```python
from build123d import *

# Parameters (mm, degrees)
SKETCH_1_W                  = 56
SKETCH_1_H                  = 62
EXTRUDE_1_DEPTH             = 82
SKETCH_4_W                  = 56
SKETCH_4_H                  = 62
SKETCH_4_R                  = 26
CUT_EXTRUDE_1_DEPTH         = 36
HOLE_WIZARD_M4_1_D          = 3.3
HOLE_WIZARD_M4_1_DEPTH      = 10.1
HOLE_WIZARD_M4_1_TIP        = 0.991420021
SKETCH_15_W                 = 23
SKETCH_15_H                 = 1.9
FILLET_1_R                  = 2
CHAMFER_2_SIZE              = 1
HOLE_WIZARD_M2_5_1_D        = 2.05
HOLE_WIZARD_M2_5_1_DEPTH    = 7.25
HOLE_WIZARD_M2_5_1_TIP      = 0.615882135
SKETCH_19_W                 = 10.5
SKETCH_19_H                 = 46
EXTRUDE_2_DEPTH             = 13
HOLE_WIZARD_M5_1_D          = 4.2
HOLE_WIZARD_M3_1_AT_2_COUNT = 2
HOLE_WIZARD_M3_1_AT_2_PITCH = 15


with BuildPart() as part:
    # 草图1 → 凸台-拉伸1 (new body)
    with BuildSketch(Plane.XY):
        with Locations((0, -3)):
            Rectangle(SKETCH_1_W, SKETCH_1_H)
    extrude(amount=EXTRUDE_1_DEPTH)

    # 草图3 → 切除-旋转2 (revolve, cut)
    with BuildSketch(Plane(origin=(0, 0, 0), x_dir=(0, 0, -1), z_dir=(1, 0, 0)), mode=Mode.PRIVATE) as cut_revolve_2_sk:
        Polygon((-82, 0), (0, 0), (0, 23), (-52, 23), (-52, 20), (-56, 20), (-56, 21), (-82, 21), align=None)
    revolve(cut_revolve_2_sk.sketch.rotate(Axis((0, 0, -5.719261836), (0, 0, 1)), 90), axis=Axis((0, 0, -5.719261836), (0, 0, 1)), mode=Mode.SUBTRACT)

    # 草图4 → 切除-拉伸1 (cut)
    with BuildSketch(Plane.XY.offset(82)):
        with Locations((0, -3)):
            Rectangle(SKETCH_4_W, SKETCH_4_H)
        Circle(SKETCH_4_R, mode=Mode.SUBTRACT)
    extrude(amount=-CUT_EXTRUDE_1_DEPTH, mode=Mode.SUBTRACT)

    # M4 螺纹孔1
    with Locations(Plane(origin=(0, 0, 0), x_dir=(-1, 0, 0), z_dir=(0, 0, -1))):
        with Locations((18.384776311, 18.384776311), (18.384776311, -18.384776311), (-18.384776311, -18.384776311), (-18.384776311, 18.384776311)):
            Hole(HOLE_WIZARD_M4_1_D / 2, depth=HOLE_WIZARD_M4_1_DEPTH)
            with Locations((0, 0, -(HOLE_WIZARD_M4_1_DEPTH + HOLE_WIZARD_M4_1_TIP / 2))):  # 118° drill point
                Cone(0, HOLE_WIZARD_M4_1_D / 2, HOLE_WIZARD_M4_1_TIP, mode=Mode.SUBTRACT)

    # 草图15 → 切除-旋转3 (revolve, cut)
    with BuildSketch(Plane(origin=(0, 0, 0), x_dir=(1, 0, 0), z_dir=(0, 1, 0))):
        with Locations((-11.5, -79.95)):
            Rectangle(SKETCH_15_W, SKETCH_15_H)
    revolve(axis=Axis((0, 0, 0), (0, 0, 1)), mode=Mode.SUBTRACT)

    # 圆角1
    fillet_1_edges = [part.edges().sort_by_distance(p)[0] for p in [
        (-26, 0, 46),
    ]]
    fillet(fillet_1_edges, radius=FILLET_1_R - 0.0001)  # a hair under: the kernel refuses the full size

    # 倒角2
    chamfer_2_edges = [part.edges().sort_by_distance(p)[0] for p in [
        (23, 0, 0),
    ]]
    chamfer(chamfer_2_edges, length=CHAMFER_2_SIZE)

    # M2.5 螺纹孔1
    with Locations(Plane(origin=(0, 28, 0), x_dir=(1, 0, 0), z_dir=(0, 1, 0))):
        with Locations((24.5, -3), (-24.5, -43.5), (-24.5, -3), (24.5, -43.5)):
            Hole(HOLE_WIZARD_M2_5_1_D / 2, depth=HOLE_WIZARD_M2_5_1_DEPTH)
            with Locations((0, 0, -(HOLE_WIZARD_M2_5_1_DEPTH + HOLE_WIZARD_M2_5_1_TIP / 2))):  # 118° drill point
                Cone(0, HOLE_WIZARD_M2_5_1_D / 2, HOLE_WIZARD_M2_5_1_TIP, mode=Mode.SUBTRACT)

    # 草图19 → 凸台-拉伸2 (add)
    with BuildSketch(Plane.XZ.offset(34)):
        with Locations((33.25, 23)):
            Rectangle(SKETCH_19_W, SKETCH_19_H)
        with Locations((-33.25, 23)):
            Rectangle(SKETCH_19_W, SKETCH_19_H)
    extrude(amount=-EXTRUDE_2_DEPTH)

    # M5 螺纹孔1 (through all)
    with Locations(Plane(origin=(0, -34, 0), x_dir=(-1, 0, 0), z_dir=(0, -1, 0))):
        with Locations((33.5, -5), (-33.5, -41), (-33.5, -5), (33.5, -41)):
            Hole(HOLE_WIZARD_M5_1_D / 2)

    # 草图24 → M3 螺纹孔1 (revolve, cut)
    with BuildSketch(Plane(origin=(28, -9, 30.5), x_dir=(0, 0, -1), z_dir=(0, 1, 0))):
        Polygon((0, 0), (0, 6.251075774), (1.25, 5.5), (1.25, 0), align=None)
    hole_wizard_m3_1 = revolve(axis=Axis((34.35, -9, 30.5), (-1, 0, 0)), mode=Mode.SUBTRACT)

    # M3 螺纹孔1 at 2: M3 螺纹孔1 ×2
    with Locations(*[(0, 0, -i * HOLE_WIZARD_M3_1_AT_2_PITCH) for i in range(1, HOLE_WIZARD_M3_1_AT_2_COUNT)]):
        add(hole_wizard_m3_1, mode=Mode.SUBTRACT)

    # 镜向1: M3 螺纹孔1 across plane
    add(hole_wizard_m3_1.mirror(Plane(origin=(0, 0, 0), x_dir=(0, 0, 1), z_dir=(1, 0, 0))), mode=Mode.SUBTRACT)

    # 镜向1 copy 1 sketch → 镜向1 copy 1 (revolve, cut)
    with BuildSketch(Plane(origin=(-28, -9, 15.5), x_dir=(0, 0, -1), z_dir=(0, 1, 0))):
        Polygon((0, 0), (0, -6.251075774), (1.25, -5.5), (1.25, 0), align=None)
    revolve(axis=Axis((-34.35, -9, 15.5), (-1, 0, 0)), mode=Mode.SUBTRACT)


solid = part.part
```
The model under review builds one solid part; all positions refer to its coordinate system, in mm. A direction names the side the tool comes from. Give positions to 0.01 mm unless a question says otherwise; leave off trailing zeros. Write each loop counter-clockwise with the first axis right and the second up, starting at its lowest first coordinate (ties: lowest second). Pieces come first, ordered by that corner, then holes. Notation, with made-up numbers: M 6.25,21.25 L 34.25,21.25 A24 cw 34.25,59.25 Z; hole C 67,14.25 d3. An arc over 180 degrees is marked long. Write item = value, one per line. Start each with the question number.
Q1. We need section B-B (z = 36.5). State the section outline as (x, y) points, plus the area to 3 significant figures.
Q2. Machinability: for faces 1 (the face through (-10, 19, 80.9)), 2 (the face through (2.994, -22.804, 26.857)), 3 (the face through (28, 3, 23)), 4 (the face through (25.288, -10.054, 29.828)), 5 (the face through (-20.03, -6.31, 67.66)), which of the approach directions +Z, -Z, +X, -X, +Y, -Y give a long, thin tool a straight path to every point of the face, cutting with its end or side? Answer none if there is none.
Q3. We need section C-C (x = 33.5). State the section outline as (y, z) points.
Q4. For line 1 (Z direction, x = -26.6, y = -9); line 2 (Z direction, x = -24.5, y = 23.5) (3 decimals); line 3 (X direction, y = -28, z = 41), list the stretches that pass through material, from the lowest coordinate up.
Q5. Clearance check with flat-ended pins moving along their axes: pin 1 (3 mm diameter, centred on y = 17, z = 39.5, fed in from +X); pin 2 (2 mm diameter, centred on x = 28.5, y = 11.5, fed in from +Z); pin 3 (5.5 mm diameter, centred on x = 33.5, z = 41, fed in from +Y). State where each tip first meets the part, or that it passes through.
Q6. Mouldability with a two-part tool opening along Z and no side actions: class faces 6 (the face through (-9, -24, 0)), 7 (the face through (-20.03, -6.31, 81.46)), 8 (the face through (31.834, -27.409, 42.278)) as released by +Z, released by -Z, zero draft, split by the parting line, or undercut.
Result set:
q1.outline = M -38.5,-34 L 38.5,-34 L 38.5,-21 L 28,-21 L 28,28 L -28,28 L -28,-21 L -38.5,-21 Z; hole C 0,0 d46
q1.area = 2,080 mm2
q2.face_1 = none
q2.face_2 = -Z
q2.face_3 = +Z, -Z, +X, +Y
q2.face_4 = +X
q2.face_5 = +Z
q3.outline = M -34,0 L -21,0 L -21,2.9 L -34,2.9 Z; M -34,7.1 L -21,7.1 L -21,38.9 L -34,38.9 Z; M -34,43.1 L -21,43.1 L -21,46 L -34,46 Z
q4.line_1 = 0 to 14.25, 16.75 to 29.25, 31.75 to 46
q4.line_2 = 0 to 1.975, 4.025 to 42.475, 44.525 to 46
q4.line_3 = -38.5 to -35.6, -31.4 to 31.4, 35.6 to 38.5
q5.pin_1 = 28
q5.pin_2 = 46
q5.pin_3 = -21
q6.face_6 = released by -Z
q6.face_7 = zero draft
q6.face_8 = undercut
